```python
from build123d import *

# Parameters (mm, degrees)
SKETCH1_W                         = 29
SKETCH1_H                         = 8
BOSS_EXTRUDE1_DEPTH               = 4
SKETCH2_W                         = 9.5
SKETCH2_H                         = 4
BOSS_EXTRUDE2_DEPTH               = 1
SKETCH3_W                         = 9.5
SKETCH3_H                         = 4
BOSS_EXTRUDE3_DEPTH               = 1
TAP_DRILL_FOR_M2_TAP1_D           = 1.6
TAP_DRILL_FOR_M2_TAP1_CSINK_D     = 1.65
TAP_DRILL_FOR_M2_TAP1_CSINK_ANGLE = 100


with BuildPart() as part:
    # Sketch1 → Boss-Extrude1 (new body)
    with BuildSketch(Plane(origin=(0, 0, 0), x_dir=(1, 0, 0), z_dir=(0, 1, 0))):
        with Locations((14.5, 4)):
            Rectangle(SKETCH1_W, SKETCH1_H)
    extrude(amount=BOSS_EXTRUDE1_DEPTH)

    # Sketch2 → Boss-Extrude2 (add)
    with BuildSketch(Plane.XY):
        with Locations((14.5, 2)):
            Rectangle(SKETCH2_W, SKETCH2_H)
    extrude(amount=BOSS_EXTRUDE2_DEPTH)

    # Sketch3 → Boss-Extrude3 (add)
    with BuildSketch(Plane(origin=(0, 0, -8), x_dir=(-1, 0, 0), z_dir=(0, 0, -1))):
        with Locations((-14.5, 2)):
            Rectangle(SKETCH3_W, SKETCH3_H)
    extrude(amount=BOSS_EXTRUDE3_DEPTH)

    # Tap Drill for M2 Tap1 (through all)
    with Locations(Plane(origin=(0, 4, 0), x_dir=(1, 0, 0), z_dir=(0, 1, 0))):
        with Locations((6.5, 4), (22.5, 4)):
            CounterSinkHole(TAP_DRILL_FOR_M2_TAP1_D / 2, TAP_DRILL_FOR_M2_TAP1_CSINK_D / 2, counter_sink_angle=TAP_DRILL_FOR_M2_TAP1_CSINK_ANGLE)


solid = part.part
```
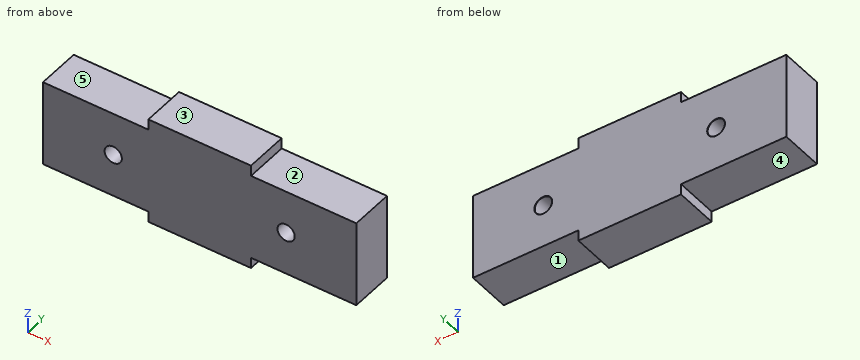
CAD build for the part. Positions are in the model's coordinates, mm. Face numbers are marked on the shaded views. A direction names the side the tool comes from. Give positions to 0.01 mm unless a question says otherwise; leave off trailing zeros. Loops run counter-clockwise (first coordinate to the right, second up) from the corner with the lowest first, then second, coordinate; pieces in that order, holes last. Notation, with made-up numbers: (79.5, 29) - (91.5, 29) arc R20 ccw to (91.5, 37) - close; hole circle Ø9 at (75, 59). An arc over 180 degrees is marked (long way). Put each result on its own line as item: value.
Q1. Slice it at B-B (z = -4). Give the cut face in (x, y) (3 decimals), plus the area to 3 significant figures.
Filled in:
outline: (0, 0) - (5.7, 0) - (5.7, 3.979) - (5.675, 4) - (0, 4) - close; (7.3, 0) - (21.7, 0) - (21.7, 3.979) - (21.675, 4) - (7.325, 4) - (7.3, 3.979) - close; (23.3, 0) - (29, 0) - (29, 4) - (23.325, 4) - (23.3, 3.979) - close
area: 103 mm²
Q2. Tool access for the marked faces 1, 2, 3, 4 and 5: list every direction of +Z, -Z, +X, -X, +Y, -Y with a clear straight run to the whole face (end or side of a thin tool).
Filled in:
face 1: -Z, +X, +Y, -Y
face 2: +Z, +X, +Y, -Y
face 3: +Z, +X, -X, +Y, -Y
face 4: -Z, -X, +Y, -Y
face 5: +Z, -X, +Y, -Y
Q3. Flat gauge pins, fed straight in: pin 1 (1 mm diameter, centred on x = 6.5, z = -4, fed in from -Y); pin 2 (1 mm diameter, centred on x = 9, y = 3.5, fed in from +Z); pin 3 (0.8 mm diameter, centred on y = 3, z = 0.5, fed in from +X); pin 4 (0.5 mm diameter, centred on y = 2.5, z = 0.5, fed in from -X). Where does each tip first touch, or does it go through?
Filled in:
pin 1: passes through
pin 2: stops at z = 0
pin 3: stops at x = 19.25
pin 4: stops at x = 9.75
Q4. Slice it at C-C (x = 9.5). Give the cut face in (y, z), plus the area to 3 significant figures.
Filled in:
outline: (0, -8) - (4, -8) - (4, 0) - (0, 0) - close
area: 32.0 mm²
Q5. Probe line 1 along X through (y, z) = (3.1, -4); line 2 along Z through (x, y) = (22.5, 2.7); line 3 along X through (y, z) = (0.7, -3.5). List the from-to ranges inside material, lowest first.
Filled in:
line 1: x = 0 to 5.7, 7.3 to 21.7, 23.3 to 29
line 2: z = -8 to -4.8, -3.2 to 0
line 3: x = 0 to 5.88, 7.12 to 21.88, 23.12 to 29
Q6. Slice it at A-A (x = 6.5). Give the cut face in (y, z) (3 decimals), plus the area to 3 significant figures.
Filled in:
outline: (0, -8) - (4, -8) - (4, -4.825) - (3.979, -4.8) - (0, -4.8) - close; (0, -3.2) - (3.979, -3.2) - (4, -3.175) - (4, 0) - (0, 0) - close
area: 25.6 mm²
